Geometry: final body of the model. Coordinates: model frame, mm. Face numbers are marked on the shaded views. A direction names the side the tool comes from. Give positions to 0.01 mm unless a question says otherwise; leave off trailing zeros. Write each loop counter-clockwise with the first axis right and the second up, starting at its lowest first coordinate (ties: lowest second). Pieces come first, ordered by that corner, then holes. Notation, with made-up numbers: M 62.25,74 L 114.25,74 A28 cw 114.25,93 Z; hole C -3.5,14 d11. An arc over 180 degrees is marked long. Use a Markdown table: item, result. Add a question column.
(1) Reachability of the marked faces 4, 5 and 6 from +Z, -Z, +X, -X, +Y, -Y: full face, straight path, thin tool, end or side. Return the list, or none.
(2) Material intervals for L1, parallel to Y at x = 24, z = -12; L2, parallel to X at y = 15.5, z = -11; L3, parallel to Z at x = 12, y = 26, sorted ascending.
(3) Pin query (flat end, axial travel): pin 1 Ø7.5 at (x, z) = (26.5, 7.5) entering from -Y; pin 2 Ø2 at (y, z) = (28, -11.5) entering from +X. Return the tip coordinate at first contact, or that it passes through.
(4) Cut plane B-B (y = 33). Output: boundary loops of the cut face in (x, z).
(5) Cut plane D-D (x = 0). Output: boundary loops of the cut face in (y, z) (3 decimals).
(6) Cut plane C-C (z = 0). Output: boundary loops of the cut face in (x, y) (3 decimals), plus the area to 3 significant figures.
(7) Draft query along X for the marked faces 1, 2 and 3. Return one class per face: released by +X, released by -X, zero draft, split by the parting line, or undercut.
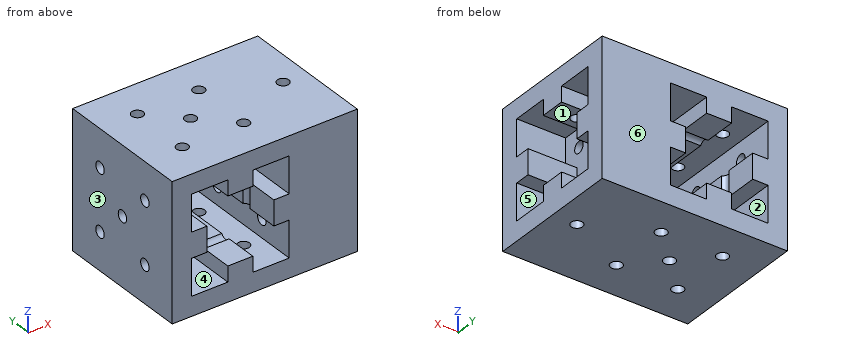
```python
from build123d import *

# Parameters (mm, degrees)
SKETCH1_W           = 35.4
SKETCH1_H           = 35.4
BOSS_EXTRUDE1_DEPTH = 35.4
SKETCH2_W           = 35.4
SKETCH2_H           = 35.4
BOSS_EXTRUDE2_DEPTH = 12.7
SKETCH5_R           = 1.5
CUT_EXTRUDE2_DEPTH  = 54.1
SKETCH6_R           = 1.5
CUT_EXTRUDE3_DEPTH  = 59.570299641


with BuildPart() as part:
    # Sketch1 → Boss-Extrude1 (new body)
    with BuildSketch(Plane(origin=(0, 0, 0), x_dir=(1, 0, 0), z_dir=(0, 1, 0))):
        Rectangle(SKETCH1_W, SKETCH1_H)
        Polygon((12.7, 3.25), (12.7, 12.7), (3.25, 12.7), (3.25, 8.7), (-3.25, 8.7), (-3.25, 12.7), (-12.7, 12.7), (-12.7, 3.25), (-8.7, 3.25), (-8.7, -3.25), (-12.7, -3.25), (-12.7, -12.7), (-3.25, -12.7), (-3.25, -8.7), (3.25, -8.7), (3.25, -12.7), (12.7, -12.7), (12.7, -3.25), (8.7, -3.25), (8.7, 3.25), align=None, mode=Mode.SUBTRACT)
    extrude(amount=BOSS_EXTRUDE1_DEPTH)

    # Sketch2 → Boss-Extrude2 (add)
    with BuildSketch(Plane(origin=(17.7, 0, 0), x_dir=(0, 0, -1), z_dir=(1, 0, 0))):
        with Locations((0, 17.7)):
            Rectangle(SKETCH2_W, SKETCH2_H)
        Polygon((12.7, 20.95), (12.7, 30.4), (3.25, 30.4), (3.25, 26.4), (-3.25, 26.4), (-3.25, 30.4), (-12.7, 30.4), (-12.7, 20.95), (-8.7, 20.95), (-8.7, 14.45), (-12.7, 14.45), (-12.7, 5), (-3.25, 5), (-3.25, 9), (3.25, 9), (3.25, 5), (12.7, 5), (12.7, 14.45), (8.7, 14.45), (8.7, 20.95), align=None, mode=Mode.SUBTRACT)
    extrude(amount=BOSS_EXTRUDE2_DEPTH)

    # Sketch5 → Cut-Extrude2 (cut, through all)
    with BuildSketch(Plane(origin=(17.7, 0, 0), x_dir=(0, 0, -1), z_dir=(1, 0, 0))):
        with Locations((0, 17.7)):
            Circle(SKETCH5_R)
        with Locations((7.975, 9.725)):
            Circle(SKETCH5_R)
        with Locations((-7.975, 9.725)):
            Circle(SKETCH5_R)
        with Locations((-7.975, 25.675)):
            Circle(SKETCH5_R)
        with Locations((7.975, 25.675)):
            Circle(SKETCH5_R)
    extrude(amount=-CUT_EXTRUDE2_DEPTH, mode=Mode.SUBTRACT)

    # Sketch6 → Cut-Extrude3 (cut, through all)
    with BuildSketch(Plane(origin=(0, 0, -17.7), x_dir=(-1, 0, 0), z_dir=(0, 0, -1))):
        with Locations((7.975, 9.725)):
            Circle(SKETCH6_R)
        with Locations((0, 17.7)):
            Circle(SKETCH6_R)
        with Locations((-7.975, 9.725)):
            Circle(SKETCH6_R)
        with Locations((-7.975, 25.675)):
            Circle(SKETCH6_R)
        with Locations((7.975, 25.675)):
            Circle(SKETCH6_R)
        with Locations((-24.05, 17.7)):
            Circle(SKETCH6_R)
    extrude(amount=-CUT_EXTRUDE3_DEPTH, mode=Mode.SUBTRACT)


solid = part.part
```
Answer list:
| question | item | result |
|---|---|---|
| 1 | face 4 | +Y, -Y |
| 1 | face 5 | +X |
| 1 | face 6 | +Z, -Z, +X, -X, +Y |
| 2 | L1 | 0 to 5, 14.45 to 16.2, 19.2 to 20.95, 30.4 to 35.4 |
| 2 | L2 | -17.7 to -12.7, -3.25 to 3.25, 12.7 to 30.4 |
| 2 | L3 | -17.7 to -12.7, -3.25 to 3.25, 12.7 to 17.7 |
| 3 | pin 1 | y = 0 |
| 3 | pin 2 | x = 17.7 |
| 4 | outline | M -17.7,-17.7 L 30.4,-17.7 L 30.4,17.7 L -17.7,17.7 Z; hole M -12.7,-12.7 L -3.25,-12.7 L -3.25,-8.7 L 3.25,-8.7 L 3.25,-12.7 L 12.7,-12.7 L 12.7,-3.25 L 8.7,-3.25 L 8.7,3.25 L 12.7,3.25 L 12.7,12.7 L 3.25,12.7 L 3.25,8.7 L -3.25,8.7 L -3.25,12.7 L -12.7,12.7 L -12.7,3.25 L -8.7,3.25 L -8.7,-3.25 L -12.7,-3.25 Z |
| 5 | outline | M 0,-17.7 L 16.2,-17.7 L 16.2,-8.7 L 11.038,-8.7 A1.5 cw 8.412,-8.7 L 0,-8.7 Z; M 0,8.7 L 8.412,8.7 A1.5 cw 11.038,8.7 L 16.2,8.7 L 16.2,17.7 L 0,17.7 Z; M 19.2,-17.7 L 35.4,-17.7 L 35.4,-8.7 L 26.988,-8.7 A1.5 cw 24.362,-8.7 L 19.2,-8.7 Z; M 19.2,8.7 L 24.362,8.7 A1.5 cw 26.988,8.7 L 35.4,8.7 L 35.4,17.7 L 19.2,17.7 Z |
| 6 | outline | M -17.7,0 L -8.7,0 L -8.7,8.412 A1.5 cw -8.7,11.038 L -8.7,16.2 L -17.7,16.2 Z; M -17.7,19.2 L -8.7,19.2 L -8.7,24.362 A1.5 cw -8.7,26.988 L -8.7,35.4 L -17.7,35.4 Z; M 8.7,0 L 30.4,0 L 30.4,9 L 17.7,9 L 17.7,16.2 L 8.7,16.2 L 8.7,11.038 A1.5 cw 8.7,8.412 Z; M 8.7,19.2 L 17.7,19.2 L 17.7,26.4 L 30.4,26.4 L 30.4,35.4 L 8.7,35.4 L 8.7,26.988 A1.5 cw 8.7,24.362 Z |
| 6 | area | 806 mm² |
| 7 | face 1 | zero draft |
| 7 | face 2 | undercut |
| 7 | face 3 | released by -X |
